Can you work these out from the model? Positions are in its coordinate system, mm. A direction names the side the tool comes from. Coordinates: 2 decimals unless noted, no trailing zeros. Order: outer loops, then holes, each group sorted by start corner. A loop starts at its lowest first (then second) coordinate and runs counter-clockwise, first axis right, second up. Notation, with made-up numbers: (89.5, -34) -> (126.5, -34) arc R18 cw to (126.5, -9) -> close; hole circle Ø6 at (87.5, -4). An arc over 180 degrees is marked (long way). Return JSON: item names as keys, results as strings. Group by question number.
1) Thinking about a two-plate mould opening in Z: for faces 1 (the cylindrical face through (-0.868, 97.121, -59.994)), 2 (the cylindrical face through (-21.207, -10.07, -42.878)), which applies, +Z half, -Z half, draft (parallel to the pull), parting line (faces both ways), or undercut?
2) If we section it at B-B, the plane x = 0: Please give me the cut outline in (y, z), then the cut area to 3 significant figures.
3) For faces 3 (the cylindrical face through (-26.53, -10.07, 39.804)), 4 (the flat face through (-29, 202, 43)), 5 (the flat face through (54.728, 97.121, -32.592)), which set-ups out of +Z, -Z, +X, -X, +Y, -Y let a thin tool reach every point of the face, with its end or its side?
4) If we section it at A-A, the plane z = 21: Please give me the cut outline in (x, y), then the cut area to 3 significant figures.
5) If I drill on probe 1 along Y at (x, z) = (-55, -22); probe 2 along X at (y, z) = (185, -54); probe 3 along X at (y, z) = (114.5, -47), over which ranges is the centre line in solid material (lowest first)? Write a range as from..to.
6) For pin 1 (2 mm diameter, centred on x = -27.5, z = 42.5, fed in from +Y); pin 2 (5 mm diameter, centred on x = -24.5, y = 120, fed in from -Z); pin 3 (6 mm diameter, centred on y = 81.5, z = -38, fed in from +X); pin 4 (4 mm diameter, centred on x = 21.5, y = 137.5, fed in from +Z), each with a flat end and sliding along its axis, tell me the tip position at first contact or that it passes through.
7) If we section it at D-D, the plane z = -13: Please give me the cut outline in (x, y), then the cut area to 3 significant figures.
8) If we section it at C-C, the plane y = 73.5: Please give me the cut outline in (x, z), then the cut area to 3 significant figures.
from build123d import *

# Parameters (mm, degrees)
BOSS_EXTRUDE1_DEPTH = 197
BOSS_EXTRUDE2_START = 15
SKETCH2_R           = 67.5
BOSS_EXTRUDE2_DEPTH = 15
SKETCH3_R           = 2.25
CUT_EXTRUDE1_DEPTH  = 10
SKETCH4_R           = 1.75
CUT_EXTRUDE2_DEPTH  = 14
MIRROR1_START       = 197
MIRROR1_OUTLINE_R   = 67.5
MIRROR1_OUTLINE_R_2 = 2.25
MIRROR1_DEPTH       = 15
MIRROR1_2_OUTLINE_R = 2.25
MIRROR1_2_DEPTH     = 5


# Read off the part's stored shape, not the designer's step: Mirror1
with BuildPart() as part:
    # Sketch1 → Boss-Extrude1 (new body)
    with BuildSketch(Plane(origin=(0, 0, 0), x_dir=(1, 0, 0), z_dir=(0, 1, 0))):
        with BuildLine():
            Line((-57.995021896, 34.537333935), (-51.551130574, 30.699852387))
            ThreePointArc((-51.551130574, 30.699852387), (0, 60), (51.551130574, 30.699852387))
            Line((51.551130574, 30.699852387), (57.995021896, 34.537333935))
            ThreePointArc((57.995021896, 34.537333935), (0, 67.5), (-57.995021896, 34.537333935))
        make_face()
    extrude(amount=BOSS_EXTRUDE1_DEPTH)

    # Sketch2 → Boss-Extrude2 (add)
    with BuildSketch(Plane.XZ.offset(BOSS_EXTRUDE2_START)):
        with Locations(Location((0, 0, 0), (0, 0, 270))):
            Circle(SKETCH2_R)
    extrude(amount=-BOSS_EXTRUDE2_DEPTH)

    # Sketch3 → Cut-Extrude1 (cut)
    with BuildSketch(Plane.XZ.offset(15)):
        with Locations(Location((22.727417579, 44.536103222, 0), (0, 0, 270))):
            Circle(SKETCH3_R)
        with Locations(Location((49.933105565, 2.585530625, 0), (0, 0, 270))):
            Circle(SKETCH3_R)
        with Locations(Location((27.205687986, -41.950572597, 0), (0, 0, 270))):
            Circle(SKETCH3_R)
        with Locations(Location((-22.727417579, -44.536103222, 0), (0, 0, 270))):
            Circle(SKETCH3_R)
        with Locations(Location((-49.933105565, -2.585530625, 0), (0, 0, 270))):
            Circle(SKETCH3_R)
        with Locations(Location((-27.205687986, 41.950572597, 0), (0, 0, 270))):
            Circle(SKETCH3_R)
    extrude(amount=-CUT_EXTRUDE1_DEPTH, mode=Mode.SUBTRACT)

    # Sketch4 → Cut-Extrude2 (cut)
    with BuildSketch(Plane.XZ.offset(5)):
        with Locations(Location((22.727417579, 44.536103222, 0), (0, 0, 270))):
            Circle(SKETCH4_R)
        with Locations(Location((49.933105565, 2.585530625, 0), (0, 0, 270))):
            Circle(SKETCH4_R)
        with Locations(Location((27.205687986, -41.950572597, 0), (0, 0, 270))):
            Circle(SKETCH4_R)
        with Locations(Location((-22.727417579, -44.536103222, 0), (0, 0, 270))):
            Circle(SKETCH4_R)
        with Locations(Location((-49.933105565, -2.585530625, 0), (0, 0, 270))):
            Circle(SKETCH4_R)
        with Locations(Location((-27.205687986, 41.950572597, 0), (0, 0, 270))):
            Circle(SKETCH4_R)
    cut_extrude2 = extrude(amount=-CUT_EXTRUDE2_DEPTH, mode=Mode.SUBTRACT)

    # Mirror1 outline → Mirror1 (add)
    with BuildSketch(Plane(origin=(0, 0, 0), x_dir=(1, 0, 0), z_dir=(0, 1, 0)).offset(MIRROR1_START)):
        Circle(MIRROR1_OUTLINE_R)
        with Locations((-27.205687986, -41.950572597)):
            Circle(MIRROR1_OUTLINE_R_2, mode=Mode.SUBTRACT)
        with Locations((22.727417579, -44.536103222)):
            Circle(MIRROR1_OUTLINE_R_2, mode=Mode.SUBTRACT)
        with Locations((49.933105565, -2.585530625)):
            Circle(MIRROR1_OUTLINE_R_2, mode=Mode.SUBTRACT)
        with Locations((-49.933105565, 2.585530625)):
            Circle(MIRROR1_OUTLINE_R_2, mode=Mode.SUBTRACT)
        with Locations((-22.727417579, 44.536103222)):
            Circle(MIRROR1_OUTLINE_R_2, mode=Mode.SUBTRACT)
        with Locations((27.205687986, 41.950572597)):
            Circle(MIRROR1_OUTLINE_R_2, mode=Mode.SUBTRACT)
    extrude(amount=MIRROR1_DEPTH)

    # Mirror1 2 outline → Mirror1 2 (add)
    with BuildSketch(Plane(origin=(0, 0, 0), x_dir=(1, 0, 0), z_dir=(0, 1, 0)).offset(MIRROR1_START)):
        with Locations((22.727417579, -44.536103222)):
            Circle(MIRROR1_2_OUTLINE_R)
        with Locations((49.933105565, -2.585530625)):
            Circle(MIRROR1_2_OUTLINE_R)
        with Locations((27.205687986, 41.950572597)):
            Circle(MIRROR1_2_OUTLINE_R)
        with Locations((-22.727417579, 44.536103222)):
            Circle(MIRROR1_2_OUTLINE_R)
        with Locations((-49.933105565, 2.585530625)):
            Circle(MIRROR1_2_OUTLINE_R)
        with Locations((-27.205687986, -41.950572597)):
            Circle(MIRROR1_2_OUTLINE_R)
    extrude(amount=MIRROR1_2_DEPTH)

    # Mirror2: Cut-Extrude2 across plane
    add(cut_extrude2.mirror(Plane.ZX.offset(98.5)), mode=Mode.SUBTRACT)


solid = part.part
Result sheet:
{
 "1": {"face 1": "+Z half", "face 2": "undercut"},
 "2": {"outline": "(-15, -67.5) -> (212, -67.5) -> (212, 67.5) -> (197, 67.5) -> (197, -60) -> (0, -60) -> (0, 67.5) -> (-15, 67.5) -> close", "area": "5,530 mm2"},
 "3": {"face 3": "-Y", "face 4": "+Y", "face 5": "+Z, +X"},
 "4": {"outline": "(-64.15, -15) -> (64.15, -15) -> (64.15, 0) -> (-64.15, 0) -> close; (-64.15, 197) -> (64.15, 197) -> (64.15, 212) -> (-64.15, 212) -> close", "area": "3,850 mm2"},
 "5": {"probe 1": "y = -15..0, 197..212", "probe 2": "x = -40.5..-26.15, 26.15..40.5", "probe 3": "x = -48.45..-37.3, 37.3..48.45"},
 "6": {"pin 1": "passes through", "pin 2": "stops at z = -63.81", "pin 3": "stops at x = 57.72", "pin 4": "stops at z = -55.21"},
 "7": {"outline": "(-66.24, -15) -> (66.24, -15) -> (66.24, 0) -> (-66.24, 0) -> close; (-66.24, 197) -> (66.24, 197) -> (66.24, 212) -> (-66.24, 212) -> close", "area": "3,970 mm2"},
 "8": {"outline": "(-58, -34.54) arc R67.5 ccw to (58, -34.54) -> (51.55, -30.7) arc R60 cw to (-51.55, -30.7) -> close", "area": "988 mm2"}
}
